```python
from build123d import *

# Parameters (mm, degrees)
SKETCH1_R                      = 6.4135
BOSS_EXTRUDE1_DEPTH            = 34.29
CUT_EXTRUDE1_REACH             = 100.106
SKETCH3_W                      = 12.7
SKETCH3_H                      = 51.6425
CUT_EXTRUDE1_DIRECTION_2_REACH = 100.106
SKETCH5_R                      = 2.159
CUT_EXTRUDE2_DEPTH             = 86.858993575
SKETCH6_W                      = 25.4
SKETCH6_H                      = 8.47980016
BOSS_EXTRUDE2_DEPTH            = 17.4625
CUT_EXTRUDE9_START             = -6.35
SKETCH12_R                     = 14.478
CUT_EXTRUDE9_DEPTH             = 15.08125
SKETCH8_R                      = 1.905
CUT_EXTRUDE11_DEPTH            = 40.9575
CUT_EXTRUDE12_START            = -4.7625
SKETCH14_R                     = 1.905
CUT_EXTRUDE12_DEPTH            = 4.7625
FILLET4_R                      = 6.35
CHAMFER1_SIZE                  = 1.5875
CUT_EXTRUDE13_DEPTH            = 95.203417847
SKETCH16_W                     = 40.857524936
SKETCH16_H                     = 6.35
BOSS_EXTRUDE3_DEPTH            = 61.16
SKETCH17_R                     = 2.159
CUT_EXTRUDE14_DEPTH            = 6.35
FILLET5_R                      = 6.35
SKETCH18_W                     = 28.157524936
SKETCH18_H                     = 38.06
BOSS_EXTRUDE4_DEPTH            = 10.8
SKETCH19_R                     = 2.1
CUT_EXTRUDE15_DEPTH            = 40
SKETCH21_R                     = 3.5
CUT_EXTRUDE16_DEPTH            = 11
SKETCH22_R                     = 3.5
CUT_EXTRUDE17_DEPTH            = 11


with BuildPart() as part:
    # Sketch1 → Boss-Extrude1 (new body)
    # profile 1 of 3: a face of its own
    with BuildSketch(Plane.XY):
        with BuildLine():
            Line((12.7, 6.75), (20.428762468, 6.75))
            ThreePointArc((20.428762468, 6.75), (31.422640825, 35.602442589), (12.7, 60.154255663))
            Line((12.7, 60.154255663), (12.7, 6.75))
        make_face()
    # profile 2 of 3: a face of its own
    with BuildSketch(Plane.XY):
        Polygon((-47, 0.4), (-10.625, 0.4), (10.625, 0.4), (47, 0.4), (47, 6.75), (12.7, 6.75), (12.7, 69.8924), (-12.7, 69.8924), (-12.7, 6.75), (-47, 6.75), align=None)
        with Locations((0, 31.0549)):
            Circle(SKETCH1_R, mode=Mode.SUBTRACT)
    # profile 3 of 3: a face of its own
    with BuildSketch(Plane.XY):
        with BuildLine():
            ThreePointArc((-12.7, 60.154255663), (-31.422640825, 35.602442589), (-20.428762468, 6.75))
            Line((-20.428762468, 6.75), (-12.7, 6.75))
            Line((-12.7, 6.75), (-12.7, 60.154255663))
        make_face()
    extrude(amount=BOSS_EXTRUDE1_DEPTH)

    # Sketch3 → Cut-Extrude1 (cut, up to next)
    with BuildSketch(Plane(origin=(12.7, 0, 0), x_dir=(0, 0, -1), z_dir=(1, 0, 0)), mode=Mode.PRIVATE) as cut_extrude1_sk1:
        with Locations((-17.145, 44.07115)):
            Rectangle(SKETCH3_W, SKETCH3_H)
    cut_extrude1_tool1 = extrude(cut_extrude1_sk1.sketch, amount=-CUT_EXTRUDE1_REACH, mode=Mode.PRIVATE) & part.part
    add(cut_extrude1_tool1.solids().sort_by_distance((12.7, 44.07115, 17.145))[0], mode=Mode.SUBTRACT)

    # Sketch3 → Cut-Extrude1 direction 2 (cut, up to next)
    with BuildSketch(Plane(origin=(12.7, 0, 0), x_dir=(0, 0, -1), z_dir=(1, 0, 0)), mode=Mode.PRIVATE) as cut_extrude1_direction_2_sk1:
        with Locations((-17.145, 44.07115)):
            Rectangle(SKETCH3_W, SKETCH3_H)
    cut_extrude1_direction_2_tool1 = extrude(cut_extrude1_direction_2_sk1.sketch, amount=CUT_EXTRUDE1_DIRECTION_2_REACH, mode=Mode.PRIVATE) & part.part
    add(cut_extrude1_direction_2_tool1.solids().sort_by_distance((12.7, 44.07115, 17.145))[0], mode=Mode.SUBTRACT)

    # Sketch5 → Cut-Extrude2 (cut, through all)
    with BuildSketch(Plane(origin=(0, 6.75, 0), x_dir=(1, 0, 0), z_dir=(0, 1, 0))):
        with Locations(Location((40, -27.94, 0), (0, 0, 180))):
            Circle(SKETCH5_R)
        with Locations(Location((40, -6.35, 0), (0, 0, 180))):
            Circle(SKETCH5_R)
        with Locations(Location((-40, -6.35, 0), (0, 0, 180))):
            Circle(SKETCH5_R)
        with Locations(Location((-40, -27.94, 0), (0, 0, 180))):
            Circle(SKETCH5_R)
    extrude(amount=-CUT_EXTRUDE2_DEPTH, mode=Mode.SUBTRACT)

    # Sketch6 → Boss-Extrude2 (add)
    with BuildSketch(Plane.XY.offset(34.29)):
        with Locations((0, 65.65249992)):
            Rectangle(SKETCH6_W, SKETCH6_H)
    boss_extrude2 = extrude(amount=BOSS_EXTRUDE2_DEPTH)

    # Sketch12 → Cut-Extrude9 (cut)
    with BuildSketch(Plane.XY.offset(23.495).offset(CUT_EXTRUDE9_START)):
        with Locations((0, 31.0549)):
            Circle(SKETCH12_R)
    cut_extrude9 = extrude(amount=CUT_EXTRUDE9_DEPTH, mode=Mode.SUBTRACT)

    # Sketch8 → Cut-Extrude11 (cut)
    with BuildSketch(Plane.XY.offset(51.7525)):
        with Locations((-4.8514, 65.65249992)):
            Circle(SKETCH8_R)
        with Locations((4.8514, 65.65249992)):
            Circle(SKETCH8_R)
    cut_extrude11 = extrude(amount=-CUT_EXTRUDE11_DEPTH, mode=Mode.SUBTRACT)

    # Sketch14 → Cut-Extrude12 (cut)
    # profile 1 of 2: a face of its own
    with BuildSketch(Plane(origin=(0, 0, 23.495), x_dir=(-1, 0, 0), z_dir=(0, 0, -1)).offset(CUT_EXTRUDE12_START)):
        Polygon((-4.8514, 60.538186898), (-0.422275, 63.095343409), (-0.422275, 68.209656431), (-3.336872358, 69.8924), (-6.365927642, 69.8924), (-9.280525, 68.209656431), (-9.280525, 63.095343409), align=None)
        with Locations(Location((-4.8514, 65.65249992, 0), (0, 0, 180))):
            Circle(SKETCH14_R, mode=Mode.SUBTRACT)
    # profile 2 of 2: a face of its own
    with BuildSketch(Plane(origin=(0, 0, 23.495), x_dir=(-1, 0, 0), z_dir=(0, 0, -1)).offset(CUT_EXTRUDE12_START)):
        Polygon((6.365927642, 69.8924), (3.336872358, 69.8924), (0.422275, 68.209656431), (0.422275, 63.095343409), (4.8514, 60.538186898), (9.280525, 63.095343409), (9.280525, 68.209656431), align=None)
        with Locations(Location((4.8514, 65.65249992, 0), (0, 0, 180))):
            Circle(SKETCH14_R, mode=Mode.SUBTRACT)
    cut_extrude12 = extrude(amount=CUT_EXTRUDE12_DEPTH, mode=Mode.SUBTRACT)

    # Mirror4: Boss-Extrude2, Cut-Extrude9, Cut-Extrude11, Cut-Extrude12 across plane
    add(boss_extrude2.mirror(Plane(origin=(0, 0, 17.145), x_dir=(1, 0, 0), z_dir=(0, 0, -1))))
    add(cut_extrude9.mirror(Plane(origin=(0, 0, 17.145), x_dir=(1, 0, 0), z_dir=(0, 0, -1))), mode=Mode.SUBTRACT)
    add(cut_extrude11.mirror(Plane(origin=(0, 0, 17.145), x_dir=(1, 0, 0), z_dir=(0, 0, -1))), mode=Mode.SUBTRACT)
    add(cut_extrude12.mirror(Plane(origin=(0, 0, 17.145), x_dir=(1, 0, 0), z_dir=(0, 0, -1))), mode=Mode.SUBTRACT)

    # Fillet4
    fillet4_edges = [part.edges().sort_by_distance(p)[0] for p in [
        (47, 3.575, 0),
        (-47, 3.575, 0),
        (-47, 3.575, 34.29),
        (47, 3.575, 34.29),
    ]]
    fillet(fillet4_edges, radius=FILLET4_R)

    # Chamfer1
    chamfer1_edges = [part.edges().sort_by_distance(p)[0] for p in [
        (-7.476567629, 43.453021652, 10.795),
    ]]
    chamfer(chamfer1_edges, length=CHAMFER1_SIZE)

    # Sketch15 → Cut-Extrude13 (cut, through all)
    with BuildSketch(Plane(origin=(0, 6.75, 0), x_dir=(1, 0, 0), z_dir=(0, 1, 0))):
        with BuildLine():
            Line((20.428762468, 1.013392391), (20.428762468, -35.303392391))
            ThreePointArc((20.428762468, -35.303392391), (22.863261605, -34.54592678), (25.4, -34.29))
            Line((25.4, -34.29), (40.65, -34.29))
            ThreePointArc((40.65, -34.29), (45.140128061, -32.430128061), (47, -27.94))
            Line((47, -27.94), (47, -6.35))
            ThreePointArc((47, -6.35), (45.140128061, -1.859871939), (40.65, 0))
            Line((40.65, 0), (25.4, 0))
            ThreePointArc((25.4, 0), (22.863261605, 0.25592678), (20.428762468, 1.013392391))
        make_face()
        with BuildLine():
            Line((-40.65, 0), (-25.4, 0))
            ThreePointArc((-25.4, 0), (-22.863261605, 0.25592678), (-20.428762468, 1.013392391))
            Line((-20.428762468, 1.013392391), (-20.428762468, -35.303392391))
            ThreePointArc((-20.428762468, -35.303392391), (-22.863261605, -34.54592678), (-25.4, -34.29))
            Line((-25.4, -34.29), (-40.65, -34.29))
            ThreePointArc((-40.65, -34.29), (-45.140128061, -32.430128061), (-47, -27.94))
            Line((-47, -27.94), (-47, -6.35))
            ThreePointArc((-47, -6.35), (-45.140128061, -1.859871939), (-40.65, 0))
        make_face()
    extrude(amount=-CUT_EXTRUDE13_DEPTH, mode=Mode.SUBTRACT)

    # Sketch16 → Boss-Extrude3 (add, symmetric)
    with BuildSketch(Plane(origin=(0, 0, 17.145), x_dir=(-1, 0, 0), z_dir=(0, 0, -1))):
        with Locations((0, 3.575)):
            Rectangle(SKETCH16_W, SKETCH16_H)
    extrude(amount=BOSS_EXTRUDE3_DEPTH, both=True)

    # Sketch17 → Cut-Extrude14 (cut)
    with BuildSketch(Plane.XZ.offset(-0.4)):
        with Locations((15.5, 57.145)):
            Circle(SKETCH17_R)
        with Locations((-15.5, 57.145)):
            Circle(SKETCH17_R)
        with Locations((15.5, -22.855)):
            Circle(SKETCH17_R)
        with Locations((-15.5, -22.855)):
            Circle(SKETCH17_R)
    extrude(amount=-CUT_EXTRUDE14_DEPTH, mode=Mode.SUBTRACT)

    # Fillet5
    fillet5_edges = [part.edges().sort_by_distance(p)[0] for p in [
        (-20.428762468, 6.75, 17.145),
        (20.428762468, 6.75, 17.145),
        (-20.428762468, 3.575, -44.015),
        (20.428762468, 3.575, -44.015),
        (-20.428762468, 3.575, 78.305),
        (20.428762468, 3.575, 78.305),
    ]]
    fillet(fillet5_edges, radius=FILLET5_R)

    # Sketch18 → Boss-Extrude4 (add)
    with BuildSketch(Plane(origin=(0, 6.75, 0), x_dir=(1, 0, 0), z_dir=(0, 1, 0))):
        with Locations((0, -59.275)):
            Rectangle(SKETCH18_W, SKETCH18_H)
    boss_extrude4 = extrude(amount=BOSS_EXTRUDE4_DEPTH)

    # Mirror5: Boss-Extrude4 across plane
    add(boss_extrude4.mirror(Plane(origin=(0, 0, 17.145), x_dir=(1, 0, 0), z_dir=(0, 0, -1))))

    # Sketch19 → Cut-Extrude15 (cut)
    with BuildSketch(Plane(origin=(0, 0, -44.015), x_dir=(-1, 0, 0), z_dir=(0, 0, -1))):
        with Locations((8.5, 12.5549)):
            Circle(SKETCH19_R)
        with Locations((-8.5, 12.5549)):
            Circle(SKETCH19_R)
    cut_extrude15 = extrude(amount=-CUT_EXTRUDE15_DEPTH, mode=Mode.SUBTRACT)

    # Mirror6: Cut-Extrude15 across plane
    add(cut_extrude15.mirror(Plane(origin=(0, 0, 17.145), x_dir=(1, 0, 0), z_dir=(0, 0, -1))), mode=Mode.SUBTRACT)

    # Sketch21 → Cut-Extrude16 (cut)
    with BuildSketch(Plane(origin=(0, 6.75, 0), x_dir=(1, 0, 0), z_dir=(0, 1, 0))):
        with Locations((15.5, -57.145)):
            Circle(SKETCH21_R)
    cut_extrude16 = extrude(amount=CUT_EXTRUDE16_DEPTH, mode=Mode.SUBTRACT)

    # Sketch22 → Cut-Extrude17 (cut)
    with BuildSketch(Plane(origin=(0, 6.75, 0), x_dir=(1, 0, 0), z_dir=(0, 1, 0))):
        with Locations((-15.5, -57.145)):
            Circle(SKETCH22_R)
    cut_extrude17 = extrude(amount=CUT_EXTRUDE17_DEPTH, mode=Mode.SUBTRACT)

    # Mirror7: Cut-Extrude16, Cut-Extrude17 across plane
    add(cut_extrude16.mirror(Plane(origin=(0, 0, 17.145), x_dir=(1, 0, 0), z_dir=(0, 0, -1))), mode=Mode.SUBTRACT)
    add(cut_extrude17.mirror(Plane(origin=(0, 0, 17.145), x_dir=(1, 0, 0), z_dir=(0, 0, -1))), mode=Mode.SUBTRACT)


solid = part.part
```
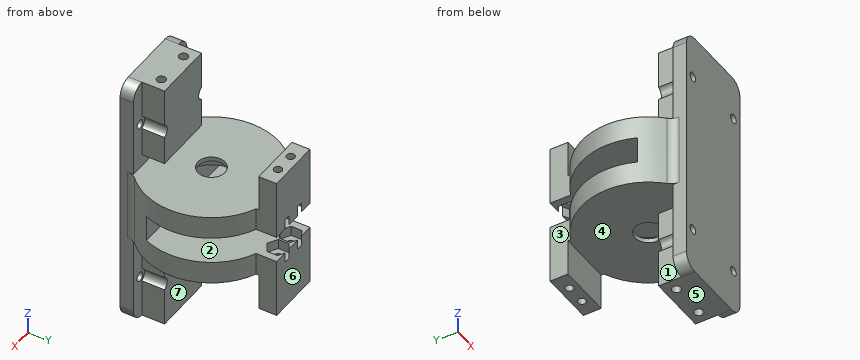
Could you check a few things on this model? Use its own coordinates, in mm. Face numbers are marked on the shaded views. A direction names the side the tool comes from. Coordinates: 2 decimals unless noted, no trailing zeros. Order: outer loops, then holes, each group sorted by start corner. A loop starts at its lowest first (then second) coordinate and runs counter-clockwise, first axis right, second up. Notation, with made-up numbers: M -8,49 L 36,49 A19 ccw 36,74 Z; hole C 74,51 d5. An arc over 180 degrees is marked long. Use a Markdown table: item, result. Add a question column.
Q1. I want a section at A-A on z = 38. Give the number of separate pieces and of enclosed holes in the cut face, then the cut area to 3 significant figures.
Q2. I want a section at C-C on z = -33.5. List the corners of the cut face in (x, y) for me, then the cut area to 3 significant figures.
Q3. Which directions (+Z, -Z, +X, -X, +Y, -Y) give clear straight access to the entire face, cutting with the end or side of a thin tool? Please do the marked faces 1, 2 and 3.
Q4. I want a section at B-B on z = 12.5. List the corners of the cut face in (x, y) for me.
Q5. If I drill on L1, parallel to Z at x = 5.5, y = 14.5 (3 decimals); L2, parallel to X at y = 64.5, z = -1; L3, parallel to Y at x = 0, z = 33, over which ranges is the centre line in solid material (lowest first)?
Q6. We'd pull the mould along Y, two halves only. Please class the marked faces 4, 5, 6 and 7: pulls with the +Y half, pulls with the -Y half, needs draft (parallel to the pull), parting line crosses it, or undercut.
Q7. I'm going to push flat-ended pins straight in: pin 1 (9.5 mm diameter, centred on x = -4, y = 65.5, fed in from +Z); pin 2 (3 mm diameter, centred on y = 10.5, z = 49.5, fed in from +X); pin 3 (8.5 mm diameter, centred on x = 6.5, z = 63, fed in from +Y). Where does each tip first touch, or does it pass through?
Checked values:
| question | item | result |
|---|---|---|
| 1 | separate pieces | 2 |
| 1 | enclosed holes | 2 |
| 1 | area | 452 mm² |
| 2 | outline | M -20.43,0.4 L 20.43,0.4 L 20.43,6.75 L 14.08,6.75 L 14.08,17.55 L -14.08,17.55 L -14.08,6.75 L -20.43,6.75 Z; hole C -8.5,12.55 d4.2; hole C 8.5,12.55 d4.2 |
| 2 | area | 536 mm² |
| 3 | face 1 | -Z, -X, +Y |
| 3 | face 2 | +X, -X, +Y |
| 3 | face 3 | +Z, -Z, -X, +Y |
| 4 | outline | M -29.05,18.25 A31.75 ccw -22.32,8.47 A6.35 cw -20.43,3.95 L -20.43,0.4 L 20.43,0.4 L 20.43,3.95 A6.35 cw 22.32,8.47 A31.75 ccw 29.05,18.25 L 6.76,18.25 A14.48 cw -6.76,18.25 Z |
| 5 | L1 | -44.015 to -5.955, 0 to 34.29, 40.245 to 78.305 |
| 5 | L2 | -12.7 to -6.37, -3.33 to 3.33, 6.37 to 12.7 |
| 5 | L3 | 0.4 to 24.64, 37.47 to 69.89 |
| 6 | face 4 | undercut |
| 6 | face 5 | needs draft |
| 6 | face 6 | pulls with the +Y half |
| 6 | face 7 | undercut |
| 7 | pin 1 | z = 51.75 |
| 7 | pin 2 | x = 14.08 |
| 7 | pin 3 | y = 17.55 |
